Geometry check sheet. Reference: the model listing, model coordinates, mm. A direction names the side the tool comes from. Round coordinates to 2 decimals unless told otherwise and drop trailing zeros. Loops run counter-clockwise (first coordinate to the right, second up) from the corner with the lowest first, then second, coordinate; pieces in that order, holes last. Notation, with made-up numbers: (-35, -22.5) - (6, -22.5) arc R20 ccw to (6, 13.5) - close; hole circle Ø2 at (-20, 69.25). An arc over 180 degrees is marked (long way). Answer in a Markdown table with one row per item. Add a question column.
```python
from build123d import *

# Parameters (mm, degrees)
EXTRUDE_1_DEPTH     = 2
SKETCH_2_R          = 5
EXTRUDE_2_DEPTH     = 2
FILLET_1_R          = 2.5
SKETCH_3_R          = 1.5
CUT_EXTRUDE_1_DEPTH = 12
SKETCH_4_R          = 1.5
CUT_EXTRUDE_2_DEPTH = 10


with BuildPart() as part:
    # 草图1 → 凸台-拉伸1 (new body)
    with BuildSketch(Plane(origin=(0, 0, 0), x_dir=(1, 0, 0), z_dir=(0, 1, 0))):
        with BuildLine():
            Line((-12.5, 40), (12.5, 40))
            ThreePointArc((12.5, 40), (14.267766953, 39.267766953), (15, 37.5))
            Line((15, 37.5), (15, 0))
            Line((15, 0), (-15, 0))
            Line((-15, 0), (-15, 37.5))
            ThreePointArc((-15, 37.5), (-14.267766953, 39.267766953), (-12.5, 40))
        make_face()
    extrude(amount=EXTRUDE_1_DEPTH)

    # 草图2 → 凸台-拉伸2 (add)
    with BuildSketch(Plane.XY):
        with BuildLine():
            Line((-15, 17), (-15, 2))
            Line((-15, 2), (15, 2))
            Line((15, 2), (15, 17))
            ThreePointArc((15, 17), (0, 32), (-15, 17))
        make_face()
        with Locations((0, 17)):
            Circle(SKETCH_2_R, mode=Mode.SUBTRACT)
    extrude(amount=-EXTRUDE_2_DEPTH)

    # 圆角1
    fillet_1_edges = [part.edges().sort_by_distance(p)[0] for p in [
        (0, 2, -2),
    ]]
    fillet(fillet_1_edges, radius=FILLET_1_R)

    # 草图3 → 切除-拉伸1 (cut)
    with BuildSketch(Plane.XZ):
        with Locations((10, -10)):
            Circle(SKETCH_3_R)
        with Locations((-10, -10)):
            Circle(SKETCH_3_R)
        with Locations((-10, -34)):
            Circle(SKETCH_3_R)
        with Locations((10, -34)):
            Circle(SKETCH_3_R)
    extrude(amount=-CUT_EXTRUDE_1_DEPTH, mode=Mode.SUBTRACT)

    # 草图4 → 切除-拉伸2 (cut)
    with BuildSketch(Plane.XY):
        with Locations((10, 17)):
            Circle(SKETCH_4_R)
        with Locations((-10, 17)):
            Circle(SKETCH_4_R)
    extrude(amount=-CUT_EXTRUDE_2_DEPTH, mode=Mode.SUBTRACT)


solid = part.part
```
Q1. Scan lines: line 1 (Z direction, x = -10, y = 0.9); line 2 (Y direction, x = 11, z = -26); line 3 (Z direction, x = 11, y = 24). Record each from-to range of solid material in increasing order. Write a range as from..to.
Q2. Release check for a two-part mould opening along Y. For faces 3 (the cylindrical face through (8.89, 18.01, -0.99)), 4 (the cylindrical face through (0.21, 2.713, -2.752)), 5 (the flat face through (-15, 1.6, -13.1)), 6 (the flat face through (0, 0, -20)) record: +Y half, -Y half, draft (parallel to the pull), parting line (faces both ways), or undercut.
Q3. Set-up check for faces 1 (the flat face through (0, 2, -22)), 2 (the flat face through (15, 1.5, -11.7)): record each of +Z, -Z, +X, -X, +Y, -Y from which the full face is reachable in a straight line by a thin tool's end or side.
Q4. Depth check by flat-ended pin: P1, Ø15, axis at x = 5, z = -16.5, coming from the +Y side; P2, Ø1, axis at x = -8, y = 4, coming from the -Z side; P3, Ø16, axis at x = 0, y = 17, coming from the -Z side. Enter the tip coordinate at first touch or a pass-through.
Q5. Cross-section at D-D, the plane x = 10. Enter the section's corners in (y, z), plus the area to 3 significant figures.
Q6. Cross-section at B-B, the plane x = 0. Enter the section's corners in (y, z), plus the area to 3 significant figures.
Q7. Cross-section at C-C, the plane z = -33. Enter the section's corners in (x, y), plus the area to 3 significant figures.
Q8. Cross-section at A-A, the plane y = 14. Enter the section's corners in (x, z).
Check sheet entries:
| question | item | result |
|---|---|---|
| 1 | line 1 | -40..-35.5, -32.5..-11.5, -8.5..0 |
| 1 | line 2 | 0..2 |
| 1 | line 3 | -2..0 |
| 2 | face 3 | undercut |
| 2 | face 4 | +Y half |
| 2 | face 5 | draft |
| 2 | face 6 | -Y half |
| 3 | face 1 | -Z, +X, -X, +Y |
| 3 | face 2 | +Z, -Z, +X, +Y, -Y |
| 4 | P1 | y = 2 |
| 4 | P2 | z = -2.21 |
| 4 | P3 | z = -2 |
| 5 | outline | (0, -40) - (2, -40) - (2, -35.5) - (0, -35.5) - close; (0, -32.5) - (2, -32.5) - (2, -11.5) - (0, -11.5) - close; (0, -8.5) - (2, -8.5) - (2, -4.5) arc R2.5 cw to (4.5, -2) - (15.5, -2) - (15.5, 0) - (0, 0) - close; (18.5, -2) - (28.18, -2) - (28.18, 0) - (18.5, 0) - close |
| 5 | area | 116 mm² |
| 6 | outline | (0, -40) - (2, -40) - (2, -4.5) arc R2.5 cw to (4.5, -2) - (12, -2) - (12, 0) - (0, 0) - close; (22, -2) - (32, -2) - (32, 0) - (22, 0) - close |
| 6 | area | 121 mm² |
| 7 | outline | (-15, 0) - (-11.12, 0) - (-11.12, 2) - (-15, 2) - close; (-8.88, 0) - (8.88, 0) - (8.88, 2) - (-8.88, 2) - close; (11.12, 0) - (15, 0) - (15, 2) - (11.12, 2) - close |
| 7 | area | 51.1 mm² |
| 8 | outline | (-15, -2) - (-4, -2) - (-4, 0) - (-15, 0) - close; (4, -2) - (15, -2) - (15, 0) - (4, 0) - close |
